from build123d import *

# Parameters (mm, degrees)
F0_W     = 90.31574
F0_H     = 50.404425
F0_R     = 11.170566
F1_DEPTH = 136.652
F2_R     = 33.726563
F3_SIZE  = 5.08


with BuildPart() as f1:
    # F0 (on Front) → F1 (new body)
    with BuildSketch(Plane.XZ):
        with Locations((-2.810655, 38.599672)):
            Rectangle(F0_W, F0_H)
        with Locations((-28.481312, 38.505986)):
            Circle(F0_R, mode=Mode.SUBTRACT)
    extrude(amount=-F1_DEPTH)

    # F2
    f2_edges = [f1.edges().sort_by_distance(p)[0] for p in [
        (42.347215, 136.652, 38.599672),
    ]]
    fillet(f2_edges, radius=F2_R)

    # F3
    f3_edges = [f1.edges().sort_by_distance(p)[0] for p in [
        (-47.968525, 136.652, 38.599672),
    ]]
    chamfer(f3_edges, length=F3_SIZE)


solid = f1.part
Could you check a few things on this model? Use its own coordinates, in mm. Round coordinates to 2 decimals unless told otherwise and drop trailing zeros. Order: outer loops, then holes, each group sorted by start corner. A loop starts at its lowest first (then second) coordinate and runs counter-clockwise, first axis right, second up.
Q1. I'm going to push a flat-ended pin straight in: P1, Ø10, axis at y = 114, z = 56.5, coming from the +X side. Where does the tip first touch, or does it pass through?
Geometry says:
P1: stops at x = 41.8
Q2. Please list where these lines run through material, in increasing order: probe 1 along Z at (x, y) = (-20.5, 49.5); probe 2 along X at (y, z) = (79, 36.5); probe 3 along X at (y, z) = (88, 35).
Geometry says:
probe 1: z = 13.4 to 30.69, 46.32 to 63.8
probe 2: x = -47.97 to -39.47, -17.49 to 42.35
probe 3: x = -47.97 to -39.09, -17.88 to 42.35
Q3. Thinking about a two-plate mould opening in X: for faces 1 (the face through (-22.476, 67.369, 47.925)), 2 (the face through (-45.46, 134.08, 38.25)), 3 (the face through (32.73, 126.51, 38.95)), 4 (the face through (-3, 67, 63.802)), which applies, released by +X, released by -X, zero draft, split by the parting line, or undercut?
Geometry says:
face 1: undercut
face 2: released by -X
face 3: released by +X
face 4: zero draft
Q4. Imagine slicing it at C-C, the plane y = 123.5. List the corners of the cut face in (x, z) for me.
Geometry says:
outline: (-47.97, 13.4) - (35.34, 13.4) - (35.34, 63.8) - (-47.97, 63.8) - close; hole circle Ø22.34 at (-28.48, 38.51)
Q5. Imagine slicing it at A-A, the plane x = -25. List the corners of the cut face in (y, z) for me, then the cut area to 3 significant figures.
Geometry says:
outline: (0, 13.4) - (136.65, 13.4) - (136.65, 27.89) - (0, 27.89) - close; (0, 49.12) - (136.65, 49.12) - (136.65, 63.8) - (0, 63.8) - close
area: 3,990 mm2
Q6. Imagine slicing it at B-B, the plane z = 29. List the corners of the cut face in (x, y) for me, then the cut area to 3 significant figures.
Geometry says:
outline: (-47.97, 0) - (-34.35, 0) - (-34.35, 136.65) - (-42.89, 136.65) - (-47.97, 131.57) - close; (-22.61, 0) - (42.35, 0) - (42.35, 102.93) arc R33.73 ccw to (8.62, 136.65) - (-22.61, 136.65) - close
area: 10,500 mm2
Q7. Imagine slicing it at D-D, the plane z = 20. List the corners of the cut face in (x, y) for me.
Geometry says:
outline: (-47.97, 0) - (42.35, 0) - (42.35, 102.93) arc R33.73 ccw to (8.62, 136.65) - (-42.89, 136.65) - (-47.97, 131.57) - close
